Verification items for the finished model (mm, model axes). Face numbers are marked on the shaded views. Coordinates: 2 decimals unless noted, no trailing zeros. Order: outer loops, then holes, each group sorted by start corner. A loop starts at its lowest first (then second) coordinate and runs counter-clockwise, first axis right, second up. Notation, with made-up numbers: (-26.5, 30.5) -> (-20.5, 30.5) arc R29 ccw to (-20.5, 54.5) -> close; hole circle Ø6 at (5.25, 45.5). An arc over 180 degrees is marked (long way). Write item = value, one per line. Start each with the question number.
1. Cross-section at C-C on x = 56.5. Record the cut outline in (y, z).
2. Cross-section at D-D on z = 41.5. Record the cut outline in (x, y), plus the area to 3 significant figures.
3. Cross-section at A-A on y = -39. Record the cut outline in (x, z).
4. Release check for a two-part mould opening along Z. For the marked faces 1 and 2 record: +Z half, -Z half, draft (parallel to the pull), parting line (faces both ways), or undercut.
5. Cross-section at B-B on z = 3. Record the cut outline in (x, y).
6. Go/stop test with flat-tipped pins: P1, Ø17, axis at x = -58.5, z = -24, coming from the -Y side; P2, Ø15.5, axis at x = -103, z = 40.5, coming from the -Y side; P3, Ø12.5, axis at y = -15, z = 24.5, coming from the -X side. Record where each tip stops, or that it passes through.
7. Thickness scan on line 1 along Z through (x, y) = (69.5, -22); line 2 along X through (y, z) = (-39.5, 4); line 3 along X through (y, z) = (-2.5, -20). Record the ranges inside material, lowest first. Write a range as from..to.
from build123d import *

# Parameters (mm, degrees)
F0_W     = 448
F0_H     = 14
F0_H_2   = 21
F1_DEPTH = 25
F2_W     = 448
F2_H     = 21
F3_DEPTH = 10
F4_W     = 50
F4_H     = 28
F5_DEPTH = 25


with BuildPart() as f1:
    # F0 (on Front) → F1 (new body)
    with BuildSketch(Plane.XZ):
        with Locations((0, 42)):
            Rectangle(F0_W, F0_H)
        with Locations((0, -42)):
            Rectangle(F0_W, F0_H)
        Polygon((-224, 0), (-224, 14), (-274, 14), (-274, 0), (-274, -14), (-224, -14), align=None)
        Polygon((274, 14), (224, 14), (224, 0), (224, -14), (274, -14), (274, 0), align=None)
        with Locations((0, 24.5)):
            Rectangle(F0_W, F0_H_2)
        Polygon((224, 0), (224, 14), (-224, 14), (-224, 0), (-224, -14), (224, -14), align=None)
        with Locations((0, -24.5)):
            Rectangle(F0_W, F0_H_2)
    extrude(amount=F1_DEPTH)

    # F2 (on face) → F3 (cut)
    with BuildSketch(Plane.XZ.offset(25)):
        Polygon((-224, 31.5), (-224, 14), (224, 14), (224, 35), (-224, 35), align=None)
        with Locations((0, -24.5)):
            Rectangle(F2_W, F2_H)
    extrude(amount=-F3_DEPTH, mode=Mode.SUBTRACT)

    # F4 (on face) → F5 (join)
    with BuildSketch(Plane.XZ.offset(25)):
        with Locations((249, 0)):
            Rectangle(F4_W, F4_H)
        with Locations((-249, 0)):
            Rectangle(F4_W, F4_H)
    extrude(amount=F5_DEPTH)


solid = f1.part
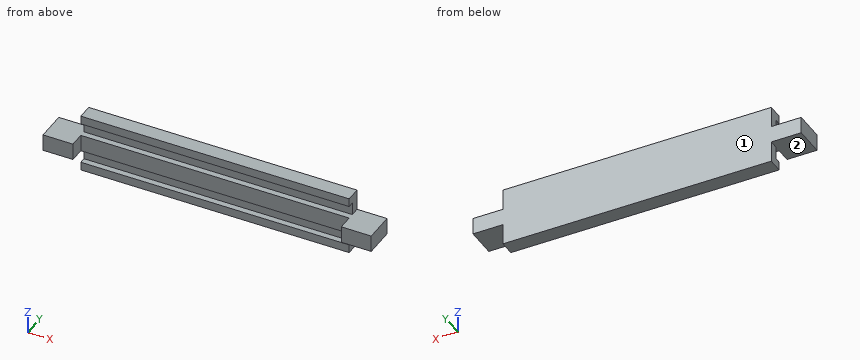
Worked out:
q1.outline = (-25, -49) -> (0, -49) -> (0, 49) -> (-25, 49) -> (-25, 35) -> (-15, 35) -> (-15, 14) -> (-25, 14) -> (-25, -14) -> (-15, -14) -> (-15, -35) -> (-25, -35) -> close
q2.outline = (-224, -25) -> (224, -25) -> (224, 0) -> (-224, 0) -> close
q2.area = 11,200 mm²
q3.outline = (-274, -14) -> (-224, -14) -> (-224, 14) -> (-274, 14) -> close; (224, -14) -> (274, -14) -> (274, 14) -> (224, 14) -> close
q4.face_1 = draft
q4.face_2 = undercut
q5.outline = (-274, -50) -> (-224, -50) -> (-224, -25) -> (224, -25) -> (224, -50) -> (274, -50) -> (274, 0) -> (-274, 0) -> close
q6.P1 = -15
q6.P2 = -25
q6.P3 = -224
q7.line_1 = -49..-35, -14..14, 35..49
q7.line_2 = -274..-224, 224..274
q7.line_3 = -224..224
